```python
from build123d import *

# Parameters (mm, degrees)
CROQUIS1_W               = 65
CROQUIS1_H               = 146
SALIENTE_EXTRUIR1_DEPTH  = 3
CROQUIS2_W               = 8
CROQUIS2_H               = 3
SALIENTE_EXTRUIR2_DEPTH  = 5
REDONDEO1_R              = 4
REDONDEO1_OF_SIMETR_A1_R = 4
CROQUIS3_W               = 2.60095456
CROQUIS3_H               = 3.001101416
SALIENTE_EXTRUIR3_DEPTH  = 0.8
REDONDEO2_R              = 2
REDONDEO2_OF_SIMETR_A5_R = 2
CROQUIS4_W               = 65
CROQUIS4_H               = 3
CROQUIS4_W_2             = 30
CROQUIS4_H_2             = 2
SALIENTE_EXTRUIR4_DEPTH  = 3
REDONDEO3_R              = 60
CROQUIS6_W               = 3.139643751
CROQUIS6_H               = 2.781946526
CORTAR_EXTRUIR1_DEPTH    = 10


# Some blends are built 0.0001 mm under size
with BuildPart() as part:
    # Croquis1 → Saliente-Extruir1 (new body)
    with BuildSketch(Plane(origin=(0, 0, 0), x_dir=(1, 0, 0), z_dir=(0, 1, 0))):
        Rectangle(CROQUIS1_W, CROQUIS1_H)
    extrude(amount=SALIENTE_EXTRUIR1_DEPTH)

    # Croquis2 → Saliente-Extruir2 (add)
    with BuildSketch(Plane(origin=(32.5, 0, 0), x_dir=(0, 0, -1), z_dir=(1, 0, 0))):
        with Locations((66, 1.5)):
            Rectangle(CROQUIS2_W, CROQUIS2_H)
    saliente_extruir2 = extrude(amount=SALIENTE_EXTRUIR2_DEPTH)

    # Redondeo1
    redondeo1_edges = [part.edges().sort_by_distance(p)[0] for p in [
        (37.5, 1.5, -62),
        (37.5, 1.5, -70),
    ]]
    fillet(redondeo1_edges, radius=REDONDEO1_R - 0.0001)  # a hair under: the kernel refuses the full size

    # Simetría1: Saliente-Extruir2 across plane
    add(saliente_extruir2.mirror(Plane(origin=(0, 0, 0), x_dir=(0, 0, 1), z_dir=(1, 0, 0))))

    # Redondeo1 of Simetría1
    redondeo1_of_simetr_a1_edges = [part.edges().sort_by_distance(p)[0] for p in [
        (-37.5, 1.5, -62),
        (-37.5, 1.5, -70),
    ]]
    fillet(redondeo1_of_simetr_a1_edges, radius=REDONDEO1_OF_SIMETR_A1_R - 0.0001)  # a hair under: the kernel refuses the full size

    # Croquis3 → Saliente-Extruir3 (add)
    with BuildSketch(Plane(origin=(32.5, 0, 0), x_dir=(0, 0, -1), z_dir=(1, 0, 0))):
        with Locations((-53.003039433, 1.500550708)):
            Rectangle(CROQUIS3_W, CROQUIS3_H)
    saliente_extruir3 = extrude(amount=SALIENTE_EXTRUIR3_DEPTH)

    # Redondeo2
    # the kernel refuses this fillet: 2 mm, written as the material it takes off along each edge
    with BuildSketch(Plane(origin=(33.3, 7.001101416, 51.702562153), x_dir=(-1, 0, 0), z_dir=(0, -1, 0)), Plane(origin=(33.3, -4, 54.303516713), x_dir=(-1, 0, 0), z_dir=(0, 1, 0))) as redondeo2_piece_1:
        with BuildLine():
            CenterArc((2, -1.6), REDONDEO2_R, 126.869897646, 53.130102354)
            Line((0, -1.6), (-0.04, -1.6))
            Line((-0.04, -1.6), (-0.04, 0))
            Line((-0.04, 0), (0, 0.04))
            ThreePointArc((0, 0.04), (0.4, 0.04), (0.776, 0.032))
            Line((0.776, 0.032), (0.8, 0))
        make_face()
    extrude(amount=11.001101416, mode=Mode.SUBTRACT)

    # Simetría5: Saliente-Extruir3 across plane
    add(saliente_extruir3.mirror(Plane(origin=(0, 0, 0), x_dir=(0, 0, 1), z_dir=(1, 0, 0))))

    # Redondeo2 of Simetría5
    # the kernel refuses this fillet: 2 mm, written as the material it takes off along each edge
    with BuildSketch(Plane(origin=(-33.3, 7.001101416, 51.702562153), x_dir=(1, 0, 0), z_dir=(0, -1, 0)), Plane(origin=(-33.3, -4, 54.303516713), x_dir=(1, 0, 0), z_dir=(0, 1, 0))) as redondeo2_of_simetr_a5_piece_1:
        with BuildLine():
            CenterArc((2, 1.6), REDONDEO2_OF_SIMETR_A5_R, 180, 53.130102354)
            Line((0, 1.6), (-0.04, 1.6))
            Line((-0.04, 1.6), (-0.04, 0))
            Line((-0.04, 0), (0, -0.04))
            ThreePointArc((0, -0.04), (0.4, -0.04), (0.776, -0.032))
            Line((0.776, -0.032), (0.8, 0))
        make_face()
    extrude(amount=11.001101416, mode=Mode.SUBTRACT)

    # Croquis4 → Saliente-Extruir4 (add)
    with BuildSketch(Plane(origin=(0, 3, 0), x_dir=(1, 0, 0), z_dir=(0, 1, 0))):
        with Locations((0, -74.5)):
            Rectangle(CROQUIS4_W, CROQUIS4_H)
        with Locations((11.5, -77)):
            Rectangle(CROQUIS4_W_2, CROQUIS4_H_2)
    extrude(amount=-SALIENTE_EXTRUIR4_DEPTH)

    # Redondeo3
    # the kernel refuses this fillet: 60 mm, written as the material it takes off along each edge
    with BuildSketch(Plane(origin=(26.5, 41.405728739, 78), x_dir=(0, 0, -1), z_dir=(0, -1, 0))) as redondeo3_piece_1:
        with BuildLine():
            CenterArc((60, -15.362291496), REDONDEO3_R, 165.164888418, 14.835111582)
            Line((0, -15.362291496), (0, 0))
            Line((0, 0), (2, 0))
        make_face()
    extrude(amount=79.811457479, mode=Mode.SUBTRACT)
    with BuildSketch(Plane(origin=(-3.5, 41.405728739, 78), x_dir=(1, 0, 0), z_dir=(0, -1, 0))) as redondeo3_piece_2:
        with BuildLine():
            CenterArc((15.362291496, -60), REDONDEO3_R, 90, 14.835111582)
            Line((0, -2), (0, 0))
            Line((0, 0), (15.362291496, 0))
        make_face()
    extrude(amount=79.811457479, mode=Mode.SUBTRACT)

    # Croquis6 → Cortar-Extruir1 (cut)
    with BuildSketch(Plane(origin=(0, 3, 0), x_dir=(1, 0, 0), z_dir=(0, 1, 0))):
        with Locations((-30.930178125, 71.609026737)):
            Rectangle(CROQUIS6_W, CROQUIS6_H)
    extrude(amount=-CORTAR_EXTRUIR1_DEPTH, mode=Mode.SUBTRACT)


solid = part.part
```
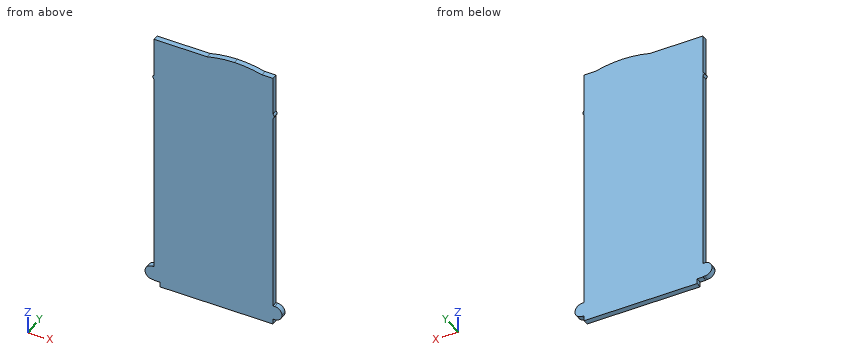
Geometry: final body of the model. Coordinates: model frame, mm. Give positions to 0.01 mm unless a question says otherwise; leave off trailing zeros. Loops run counter-clockwise (first coordinate to the right, second up) from the corner with the lowest first, then second, coordinate; pieces in that order, holes last. Notation, with made-up numbers: (47.5, 33) -> (91.5, 33) arc R18 cw to (91.5, 51) -> close; hole circle Ø9 at (64.5, -22.75). An arc over 180 degrees is marked (long way). Use CSV: the item, a comma, the result in double quotes.
(1) First-contact query: P1, Ø0.8, axis at x = -33, y = 1, coming from the +Z side; P2, Ø1.5, axis at y = 1.5, z = -3, coming from the -X side; P3, Ø1.5, axis at y = 1, z = 69.5, coming from the +X side; P4, Ø1.1, axis at x = 33, y = 2, coming from the -Z side. Flat tips, straight axial feed; report the tip coordinate or a pass-through.
From the geometry:
P1,"z = 54.22"
P2,"x = -32.5"
P3,"x = 32.5"
P4,"z = -73"
(2) Cut plane B-B (z = 37). Output: boundary loops of the cut face in (x, y), plus the area to 3 significant figures.
From the geometry:
outline,"(-32.5, 0) -> (32.5, 0) -> (32.5, 3) -> (-32.5, 3) -> close"
area,"195 mm^2"
(3) Ray query, line 1 along Z through (x, y) = (-29, 2.05); line 2 along X through (y, z) = (2.5, -37.5); line 3 along Y through (x, z) = (-3.5, -17). Return the intervals inside material, ascending. Write a range as [from, to].
From the geometry:
line 1,"[-73, 76]"
line 2,"[-32.5, 32.5]"
line 3,"[0, 3]"
